```python
from build123d import *

# Parameters (mm, degrees)
BOSS_EXTRUDE1_DEPTH = 390
CUT_EXTRUDE2_DEPTH  = 14
CUT_EXTRUDE3_DEPTH  = 50
BOSS_EXTRUDE2_DEPTH = 10
BOSS_EXTRUDE4_START = 22
BOSS_EXTRUDE4_DEPTH = 78
SKETCH22_R          = 2.1
CUT_EXTRUDE4_DEPTH  = 15
SKETCH23_R          = 3.1
CUT_EXTRUDE5_DEPTH  = 60
SKETCH24_W          = 17
SKETCH24_H          = 210
CUT_EXTRUDE6_DEPTH  = 414.617211155


with BuildPart() as part:
    # Sketch1 → Boss-Extrude1 (new body)
    with BuildSketch(Plane(origin=(0, 0, 0), x_dir=(1, 0, 0), z_dir=(0, 1, 0))):
        with BuildLine():
            Line((-10, -5.773502692), (-86.602540378, -50))
            Line((-86.602540378, -50), (-79.102540378, -62.990381057))
            Line((-79.102540378, -62.990381057), (-53.121778265, -47.990381057))
            Line((-53.121778265, -47.990381057), (-50.621778265, -52.320508076))
            Line((-50.621778265, -52.320508076), (-76.602540378, -67.320508076))
            Line((-76.602540378, -67.320508076), (-66.602540378, -84.641016151))
            Line((-66.602540378, -84.641016151), (0, -46.188021535))
            Line((0, -46.188021535), (66.602540378, -84.641016151))
            Line((66.602540378, -84.641016151), (76.602540378, -67.320508076))
            Line((76.602540378, -67.320508076), (50.621778265, -52.320508076))
            Line((50.621778265, -52.320508076), (53.121778265, -47.990381057))
            Line((53.121778265, -47.990381057), (79.102540378, -62.990381057))
            Line((79.102540378, -62.990381057), (86.602540378, -50))
            Line((86.602540378, -50), (10, -5.773502692))
            ThreePointArc((10, -5.773502692), (0, -3.094010768), (-10, -5.773502692))
        make_face()
    extrude(amount=BOSS_EXTRUDE1_DEPTH)

    # Sketch18 → Cut-Extrude2 (cut)
    with BuildSketch(Plane.XZ):
        Polygon((-76.602540378, 67.320508076), (0, 23.094010768), (76.602540378, 67.320508076), (66.602540378, 84.641016151), (0, 46.188021535), (-66.602540378, 84.641016151), align=None)
    extrude(amount=-CUT_EXTRUDE2_DEPTH, mode=Mode.SUBTRACT)

    # Sketch19 → Cut-Extrude3 (cut)
    with BuildSketch(Plane(origin=(0, 390, 0), x_dir=(1, 0, 0), z_dir=(0, 1, 0))):
        Polygon((76.602540378, -67.320508076), (0, -23.094010768), (-76.602540378, -67.320508076), (-79.102540378, -62.990381057), (0, -17.320508076), (79.102540378, -62.990381057), align=None)
    extrude(amount=-CUT_EXTRUDE3_DEPTH, mode=Mode.SUBTRACT)

    # Sketch20 → Boss-Extrude2 (add)
    with BuildSketch(Plane.XZ):
        Polygon((76.602540378, 67.320508076), (50.621778265, 52.320508076), (53.121778265, 47.990381057), (79.102540378, 62.990381057), align=None)
        Polygon((-50.621778265, 52.320508076), (-76.602540378, 67.320508076), (-79.102540378, 62.990381057), (-53.121778265, 47.990381057), align=None)
    extrude(amount=-BOSS_EXTRUDE2_DEPTH)

    # Boss-Extrude3: read off the stored shape, not the designer's step
    # Boss-Extrude3: loft between two sections, ruled curve by curve
    boss_extrude3_from = [
        Edge.make_line((-53.612159322, 357.320508076, 107.141016151), (0, 357.320508076, 76.188021535)),
        Edge.make_line((-53.612159322, 368.206188758, 107.141016151), (0, 368.206188758, 76.188021535)),
        Edge.make_line((0, 368.206188758, 76.188021535), (0, 357.320508076, 76.188021535)),
        Edge.make_line((-53.612159322, 368.206188758, 107.141016151), (-53.612159322, 357.320508076, 107.141016151)),
    ]
    boss_extrude3_to = [
        Edge.make_line((-66.602540378, 340, 84.641016151), (0, 340, 46.188021535)),
        Edge.make_line((-66.602540378, 375, 84.641016151), (0, 375, 46.188021535)),
        Edge.make_line((0, 375, 46.188021535), (0, 340, 46.188021535)),
        Edge.make_line((-66.602540378, 375, 84.641016151), (-66.602540378, 340, 84.641016151)),
    ]
    boss_extrude3 = Solid(Shell([*[Face.make_surface_from_curves(boss_extrude3_from[k], boss_extrude3_to[k]) for k in range(4)], Face(Wire(boss_extrude3_from)), Face(Wire(boss_extrude3_to))]))
    add(boss_extrude3)

    # Boss-Extrude4: read off the stored shape, not the designer's step
    # Boss-Extrude4 outline → Boss-Extrude4 (add)
    with BuildSketch(Plane(origin=(0, 0, 0), x_dir=(0.49999999999999767, 0, -0.86602540378444), z_dir=(0.8660254037844399, 0, 0.49999999999999795)).offset(BOSS_EXTRUDE4_START)):
        Polygon((-65.980762114, 357.320508076), (-40, 340), (-40, 375), (-65.980762114, 368.206188758), align=None)
    extrude(amount=BOSS_EXTRUDE4_DEPTH)

    # Sketch22 → Cut-Extrude4 (cut)
    with BuildSketch(Plane(origin=(47.172106066, 360.789319124, 81.704484407), x_dir=(0.9919674102096397, -0.12336978823439819, -0.027938368473838713), z_dir=(0.12649370372465277, 0.9674695714450555, 0.21909352168866236))):
        with Locations(Location((-89.639756751, -1.109544744, 0), (0, 0, 270))):
            Circle(SKETCH22_R)
    cut_extrude4 = extrude(amount=-CUT_EXTRUDE4_DEPTH, mode=Mode.SUBTRACT)

    # Mirror1: Cut-Extrude4 across plane
    add(cut_extrude4.mirror(Plane(origin=(0, 0, 0), x_dir=(0, 0, 1), z_dir=(1, 0, 0))), mode=Mode.SUBTRACT)

    # Sketch23 → Cut-Extrude5 (cut)
    with BuildSketch(Plane.XZ.offset(-14)):
        with Locations(Location((-25.980762114, 49.641016151, 0), (0, 0, 270))):
            Circle(SKETCH23_R)
        with Locations(Location((-51.961524227, 64.641016151, 0), (0, 0, 270))):
            Circle(SKETCH23_R)
    cut_extrude5 = extrude(amount=-CUT_EXTRUDE5_DEPTH, mode=Mode.SUBTRACT)

    # Mirror2: Cut-Extrude5 across plane
    add(cut_extrude5.mirror(Plane(origin=(0, 0, 0), x_dir=(0, 0, 1), z_dir=(1, 0, 0))), mode=Mode.SUBTRACT)

    # Sketch24 → Cut-Extrude6 (cut, through all)
    with BuildSketch(Plane(origin=(0, 0, 0), x_dir=(-0.8660254037844417, 0, -0.4999999999999947), z_dir=(0.4999999999999947, 0, -0.8660254037844417))):
        with Locations((-91.5, 119)):
            Rectangle(SKETCH24_W, SKETCH24_H)
    extrude(amount=-CUT_EXTRUDE6_DEPTH, mode=Mode.SUBTRACT)


solid = part.part
```
Input: part model. Units: mm. Frame: model coordinates. A direction names the side the tool comes from. Give positions to 0.01 mm unless a question says otherwise; leave off trailing zeros. Order: outer loops, then holes, each group sorted by start corner. A loop starts at its lowest first (then second) coordinate and runs counter-clockwise, first axis right, second up. Notation, with made-up numbers: M 26,43 L 84,43 A25 cw 84,73 Z; hole C 50.5,89.5 d7. An arc over 180 degrees is marked long. Return JSON: item names as keys, results as strings.
1) Contact query for flat-ended pins moving along their axis: pin 1 (6 mm diameter, centred on x = -38, z = 72, fed in from +Y); pin 2 (8 mm diameter, centred on x = -14.5, y = 174, fed in from +Z); pin 3 (8 mm diameter, centred on x = 25.98, z = 49.64, fed in from -Y); pin 4 (4 mm diameter, centred on x = 46, z = 34.5, fed in from -Y). Output: stop coordinate, or through.
Taken from the geometry:
{"pin 1": "stops at y = 374.91", "pin 2": "stops at z = 56.87", "pin 3": "stops at y = 14", "pin 4": "stops at y = 0"}
2) Section query B-B on x = 35. Output: boundary loops of the cut face in (y, z), and give its area (3 significant figures).
Taken from the geometry:
{"outline": "M 0,20.21 L 390,20.21 L 390,37.53 L 340,37.53 L 340,43.3 L 390,43.3 L 390,66.4 L 375,66.4 L 368.21,96.4 L 357.32,96.4 L 340,66.4 L 14,66.4 L 14,43.3 L 0,43.3 Z", "area": "18,100 mm2"}
3) Access query for faces 1 (the face through (-33.767, 174.718, 65.684)), 2 (the face through (8, 340, 27)), 3 (the face through (26.431, 362.84, 91.448)), 4 (the face through (-33.767, 382.395, 65.684)). Directions: +Z, -Z, +X, -X, +Y, -Y. A direction counts if a zero-diameter tool reaches every point of the face in a straight line with its end or side. Return the directions, or none.
Taken from the geometry:
{"face 1": "+Z, -Y", "face 2": "+Y", "face 3": "+Z, +Y, -Y", "face 4": "+Z, +Y"}
4) Mould query, pull axis Y, two halves, no side actions, for faces 5 (the face through (-43.95, 364.97, 82.08)), 6 (the face through (32.84, 382.4, 65.15)), 7 (the face through (26.43, 371.65, 76.24)), 8 (the face through (76, 14, 52)). Classes: released by +Y, released by -Y, zero draft, split by the parting line, or undercut.
Taken from the geometry:
{"face 5": "undercut", "face 6": "zero draft", "face 7": "released by +Y", "face 8": "undercut"}
5) Section query D-D on y = 260. Output: boundary loops of the cut face in (x, z).
Taken from the geometry:
{"outline": "M -86.6,50 L -10,5.77 A20 ccw 10,5.77 L 86.6,50 L 79.1,62.99 L 53.12,47.99 L 50.62,52.32 L 76.6,67.32 L 66.6,84.64 L 0,46.19 L -66.6,84.64 L -76.6,67.32 L -50.62,52.32 L -53.12,47.99 L -79.1,62.99 Z"}
6) Section query C-C on z = 31. Output: boundary loops of the cut face in (x, y), and give its area (3 significant figures).
Taken from the geometry:
{"outline": "M -53.69,0 L -13.69,0 L -13.69,14 L 13.69,14 L 13.69,0 L 53.69,0 L 53.69,390 L 23.69,390 L 23.69,340 L 13.69,340 L 13.69,390 L -13.69,390 L -13.69,340 L -23.69,340 L -23.69,390 L -53.69,390 Z", "area": "40,500 mm2"}
7) Section query A-A on y = 136. Output: boundary loops of the cut face in (x, z), and give its area (3 significant figures).
Taken from the geometry:
{"outline": "M -86.6,50 L -10,5.77 A20 ccw 10,5.77 L 71.88,41.5 L 64.38,54.49 L 53.12,47.99 L 50.62,52.32 L 61.88,58.82 L 51.88,76.14 L 0,46.19 L -66.6,84.64 L -76.6,67.32 L -50.62,52.32 L -53.12,47.99 L -79.1,62.99 Z", "area": "6,160 mm2"}
8) Line query: L1, parallel to X at y = 105.5, z = 56.5; L2, parallel to X at y = 77, z = 52.5; L3, parallel to X at y = 57.5, z = 51.5. Output: solid intervals per line, ascending. Write a range as [from, to].
Taken from the geometry:
{"L1": "x = [-82.85, -67.86], [-57.86, -17.86], [17.86, 57.86]", "L2": "x = [-85.16, -60.93], [-50.93, -10.93], [10.93, 50.93], [60.93, 65.53]", "L3": "x = [-85.74, -59.2], [-51.1, -28.46], [-23.5, -9.2], [9.2, 23.5], [28.46, 51.1], [59.2, 66.11]"}
